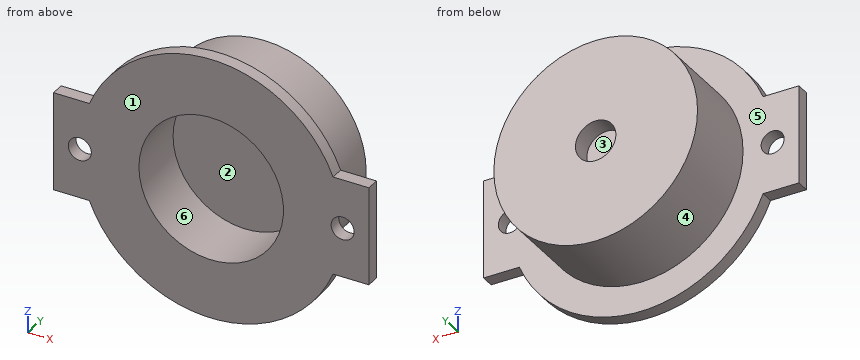
Autodesk Inventor part; units mm, degrees
ref_plane "YZ Plane" through (0, 0, 0) normal (1, 0, 0) x (0, 1, 0)
ref_plane "XZ Plane" through (0, 0, 0) normal (0, 1, 0) x (-1, 0, 0)
ref_plane "XY Plane" through (0, 0, 0) normal (0, 0, 1) x (1, 0, 0)
sketch "Sketch1" plane through (0, 0, 0) normal (0, 1, 0) x (-1, 0, 0)
  circle A0 centre (0, 0) radius 1.5
  circle A1 centre (0, 0) radius 20
  line L0 (24, -7.5) -> (-24, -7.5)
  line L1 (-24, -7.5) -> (-24, 7.5)
  line L2 (-24, 7.5) -> (24, 7.5)
  line L3 (24, 7.5) -> (24, -7.5)
  line L4 (24, -7.5) -> (-24, 7.5) construction
  line L5 (-24, -7.5) -> (24, 7.5) construction
  circle A2 centre (0, 0) radius 11
  circle A3 centre (20, 0) radius 1.75
  circle A4 centre (-20, 0) radius 1.75
  circle A5 centre (0, 0) radius 15.5
  point P0 (-18.5405, -7.5)
  point P1 (18.5405, -7.5)
  point P2 (18.5405, 7.5)
  point P3 (-18.5405, 7.5)
  dimension "d0" = 40
  dimension "d1" = 48
  dimension "d2" = 15
  dimension "d3" = 22
  dimension "d4" = 3.5
  dimension "d5" = 3.5
  dimension "d6" = 31
extrude "Extrusion1" add sketch "Sketch1" along normal blind 2 contours A3 A1 L0 A5 L2 | A1 L2 L3 L0 A3 | L2 A5 A1 | A1 L0 A5 | L2 A5 L0 A1 A4 | A1 A4 L0 L1 L2
extrude "Extrusion2" add sketch "Sketch1" along normal blind 9 contours A5 L0 A2 L2 | L2 A2 A5 | A5 L0 A2 | L2 A2 L0 A5
sketch "Sketch2" plane through (0, 9, 0) normal (0, 1, 0) x (1, 0, 0)
  circle A0 centre (0, 0) radius 15.5
  circle A1 centre (0, 0) radius 8.3846
  circle A2 centre (0, 0) radius 3.075
  dimension "d11" = 31
  dimension "d12" = 6.15
extrude "Extrusion3" add sketch "Sketch2" along normal blind 5 contours A0 | A1
extrude "Extrusion4" add sketch "Sketch2" along normal blind 2 contours A1 | A2
properties part number "magnetholder"
CAD build for the part. Positions are in the model's coordinates, mm. Face numbers are marked on the shaded views. A direction names the side the tool comes from. Give positions to 0.01 mm unless a question says otherwise; leave off trailing zeros. Loops run counter-clockwise (first coordinate to the right, second up) from the corner with the lowest first, then second, coordinate; pieces in that order, holes last. Notation, with made-up numbers: M 20.25,3.5 L 51.25,3.5 A11 ccw 51.25,23.5 Z; hole C -13,-38 d7. An arc over 180 degrees is marked long. Answer in a Markdown table with one row per item. Add a question column.
Item 1: Drop flat-ended pins along their axis: P1, Ø11, axis at x = 1, z = 2.5, coming from the -Y side; P2, Ø1.6, axis at x = 20.5, y = 0.5, coming from the +Z side; P3, Ø1, axis at x = -5, y = 7, coming from the -Z side. Give the stop position or say it passes through.
Item 2: Mould opens along X. For the marked faces 4, 5 and 6 say: +X half, -X half, draft (parallel to the pull), parting line (faces both ways), or undercut.
Item 3: Band-saw the part on C-C on z = 17.5. Give the cut face in (x, y).
Item 4: Tool access for the marked faces 1, 2 and 3: list every direction of +Z, -Z, +X, -X, +Y, -Y with a clear straight run to the whole face (end or side of a thin tool).
Item 5: Band-saw the part on D-D on x = -17.5. Give the cut face in (y, z).
Item 6: Probe probe 1 along X at (y, z) = (0.75, 0); probe 2 along Z at (x, y) = (-20, 0.55); probe 3 along Z at (x, y) = (0, 12.7) (3 decimals). List the from-to ranges inside material, lowest first.
Item 7: Band-saw the part on B-B on y = 7.25. Give the cut face in (x, z).
Item 8: Band-saw the part on A-A on x = 20. Give the cut face in (y, z), then the cut area to 3 significant figures.
Reply:
| question | item | result |
|---|---|---|
| 1 | P1 | stops at y = 9 |
| 1 | P2 | stops at z = 7.5 |
| 1 | P3 | stops at z = -14.83 |
| 2 | face 4 | parting line |
| 2 | face 5 | draft |
| 2 | face 6 | undercut |
| 3 | outline | M -9.68,0 L 9.68,0 L 9.68,2 L -9.68,2 Z |
| 4 | face 1 | +Z, -Z, +X, -X, -Y |
| 4 | face 2 | -Y |
| 4 | face 3 | +Y |
| 5 | outline | M 0,-9.68 L 2,-9.68 L 2,9.68 L 0,9.68 Z |
| 6 | probe 1 | x = -24 to -21.75, -18.25 to -11, 11 to 18.25, 21.75 to 24 |
| 6 | probe 2 | z = -7.5 to -1.75, 1.75 to 7.5 |
| 6 | probe 3 | z = -15.5 to -3.075, 3.075 to 15.5 |
| 7 | outline | C 0,0 d31; hole C 0,0 d22 |
| 8 | outline | M 0,-7.5 L 2,-7.5 L 2,-1.75 L 0,-1.75 Z; M 0,1.75 L 2,1.75 L 2,7.5 L 0,7.5 Z |
| 8 | area | 23.0 mm^2 |
